Geometry: final body of the model. Coordinates: model frame, mm. Face numbers are marked on the shaded views. A direction names the side the tool comes from. Give positions to 0.01 mm unless a question says otherwise; leave off trailing zeros. Write each loop counter-clockwise with the first axis right and the second up, starting at its lowest first coordinate (ties: lowest second). Pieces come first, ordered by that corner, then holes.
Q1. Cut plane A-A on x = 14.5. Return the cut outline in (y, z).
Q2. Cut plane C-C on z = 84. Return the cut outline in (x, y), plus the area to 3 significant figures.
Q3. Reachability of the marked faces 1, 2 and 3 from +Z, -Z, +X, -X, +Y, -Y: full face, straight path, thin tool, end or side. Return the list, or none.
Q4. Line query: L1, parallel to X at y = -16, z = 141; L2, parallel to Z at x = 14, y = -18.5; L3, parallel to X at y = -46, z = 16. Output: solid intervals per line, ascending.
Q5. Cut plane B-B on y = -27. Return the cut outline in (x, z), plus the area to 3 significant figures.
Q6. Draft query along X for the marked faces 4, 5 and 6. Return one class per face: pulls with the +X half, pulls with the -X half, needs draft (parallel to the pull), parting line crosses it, or undercut.
Q7. Pin query (flat end, axial travel): pin 1 (1.5 mm diameter, centred on y = -38.5, z = 67, fed in from +X); pin 2 (23 mm diameter, centred on y = -26.5, z = 120.5, fed in from -X); pin 3 (6 mm diameter, centred on y = -45, z = 47, fed in from -X); pin 4 (4 mm diameter, centred on x = 0.5, z = 100.5, fed in from -Y). Return the tip coordinate at first contact, or that it passes through.
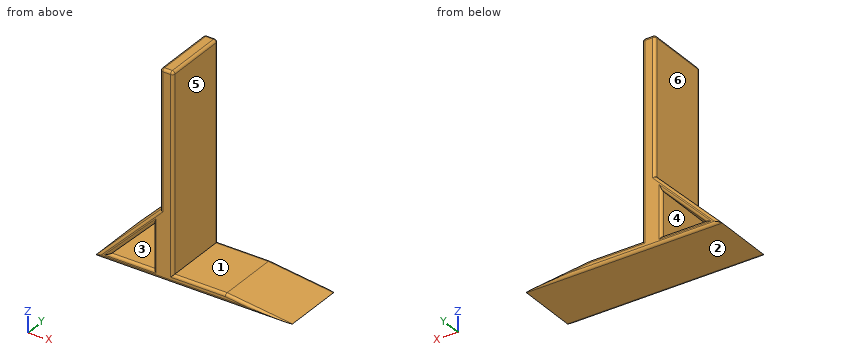
```python
from build123d import *

# Parameters (mm, degrees)
F1_DEPTH = 50
F2_R     = 2


with BuildPart() as f1:
    # F0 (on Front) → F1 (new body)
    with BuildSketch(Plane.XZ):
        Polygon((0, 45), (0, 0), (10, 0), (10, 150), (0, 150), align=None)
        Polygon((0, -6), (0, 0), (0, 45), (-50, -6), align=None)
        Polygon((-5, 32.757872), (-5, -1), (-38.095953, -1), align=None, mode=Mode.SUBTRACT)
        Polygon((10, 0), (0, 0), (0, -6), (100, -6), (50, 0), align=None)
    extrude(amount=F1_DEPTH)

    # F2
    f2_edges = [f1.edges().sort_by_distance(p)[0] for p in [
        (0, -50, 97.5),
        (-25, -50, 19.5),
        (25, -50, -6),
        (75, -50, -3),
        (30, -50, 0),
        (10, -50, 75),
        (5, -50, 150),
        (-21.547976, -50, -1),
        (-21.547976, -50, 15.878936),
        (-5, -50, 15.878936),
        (10, 0, 75),
        (5, 0, 150),
        (0, 0, 97.5),
        (-25, 0, 19.5),
        (25, 0, -6),
        (75, 0, -3),
        (30, 0, 0),
        (-21.547976, 0, -1),
        (-21.547976, 0, 15.878936),
        (-5, 0, 15.878936),
        (10, -25, 150),
        (0, -25, 150),
    ]]
    fillet(f2_edges, radius=F2_R)


solid = f1.part
```
Data:
1. outline: (-50, -4) arc R2 ccw to (-48, -6) - (-2, -6) arc R2 ccw to (0, -4) - (0, -2) arc R2 ccw to (-2, 0) - (-48, 0) arc R2 ccw to (-50, -2) - close
2. outline: (0, -48) arc R2 ccw to (2, -50) - (8, -50) arc R2 ccw to (10, -48) - (10, -2) arc R2 ccw to (8, 0) - (2, 0) arc R2 ccw to (0, -2) - close
2. area: 497 mm2
3. face 1: +Z, +X, +Y, -Y
3. face 2: -Z, +X, -X, +Y, -Y
3. face 3: +Y, -Y
4. L1: x = 0 to 10
4. L2: z = -6 to 0
4. L3: x = -28.43 to -21.43, -5 to 10
5. outline: (-50, -6) - (100, -6) - (50, 0) - (10, 0) - (10, 148) arc R2 ccw to (8, 150) - (2, 150) arc R2 ccw to (0, 148) - (0, 45) - close; hole (-38.1, -1) - (-5, -1) - (-5, 32.76) - close
5. area: 2,660 mm2
6. face 4: undercut
6. face 5: pulls with the +X half
6. face 6: pulls with the -X half
7. pin 1: stops at x = 10
7. pin 2: stops at x = 0
7. pin 3: stops at x = -0.98
7. pin 4: stops at y = -50
